Check sheet for the modelled part. Datum: model origin and axes. Units: mm. A direction names the side the tool comes from. Give positions to 0.01 mm unless a question says otherwise; leave off trailing zeros. Order: outer loops, then holes, each group sorted by start corner. A loop starts at its lowest first (then second) coordinate and runs counter-clockwise, first axis right, second up.
Item 1: Sectioned sample at D-D on z = 49. Record the boundary of the cut face in (x, y), and give its area (3 significant figures).
Item 2: Material ranges on line 1 along X through (y, z) = (-24.5, 8); line 2 along Z through (x, y) = (34, -23); line 3 along Z through (x, y) = (18, -21.5), recorded low to high.
Item 3: Gauge pin test, flat ends, axial feed: P1, Ø10, axis at y = -17, z = 9.5, coming from the -X side; P2, Ø6.5, axis at y = -19, z = 34.5, coming from the +X side; P3, Ø5.5, axis at y = -20, z = -6, coming from the -X side; P4, Ø4.5, axis at y = -20.5, z = 8, coming from the -X side. Record the tip position at first contact, or that the pin passes through.
Item 4: Sectioned sample at A-A on z = 9. Record the boundary of the cut face in (x, y), and give its area (3 significant figures).
Item 5: Sectioned sample at B-B on y = -9.5. Record the boundary of the cut face in (x, z), and give its area (3 significant figures).
Item 6: Access from +Z, -Z, +X, -X, +Y, -Y to the whole of each face (thin tool, end or side, straight path). Record for faces 4 (the flat face through (65.827, -19, 27)), 5 (the flat face through (15, -19, 22.991)), 6 (the flat face through (14.111, -19, 1)), 7 (the flat face through (49, -19, 40.581)).
Item 7: Sectioned sample at C-C on x = 49. Record the boundary of the cut face in (y, z).
Item 8: Release check for a two-part mould opening along Z. For faces 1 (the flat face through (40, -6, -15.82)), 2 (the flat face through (31, -19, 40.581)), 3 (the flat face through (52.509, -19, 1)) record: released by +Z, released by -Z, zero draft, split by the parting line, or undercut.
from build123d import *

# Parameters (mm, degrees)
F1_DEPTH = 25.4
F3_DEPTH = 12.7
F4_R     = 3.048


with BuildPart() as f1:
    # F0 (on Front) → F1 (new body)
    with BuildSketch(Plane.XZ):
        Polygon((65.826714, 50.568782), (14.111398, 50.568782), (14.111398, 36.474694), (27.428646, 36.474694), (27.428646, 40.580846), (34.53118, 40.580846), (34.53118, 19.051294), (24.432266, 19.051294), (24.432266, 22.990979), (27.428646, 22.990979), (27.428646, 30.481933), (14.111398, 30.481933), (14.111398, 22.990979), (16.885825, 22.990979), (16.885825, 4.957206), (14.111398, 4.957206), (14.111398, -2.81119), (27.428646, -2.81119), (27.428646, 4.846229), (24.432266, 4.957206), (24.432266, 10.284104), (34.53118, 10.284104), (34.53118, -2.478259), (32.422613, -2.478259), (32.422613, -9.469814), (47.515498, -9.469814), (47.515498, -2.478259), (45.406932, -2.478259), (45.406932, 10.284104), (55.505846, 10.284104), (55.505846, 4.957206), (52.509466, 4.846229), (52.509466, -2.81119), (65.826714, -2.81119), (65.826714, 4.957206), (63.052287, 4.957206), (63.052287, 22.990979), (65.826714, 22.990979), (65.826714, 30.481933), (52.509466, 30.481933), (52.509466, 22.990979), (55.505846, 22.990979), (55.505846, 19.051294), (45.406932, 19.051294), (45.406932, 40.580846), (52.509466, 40.580846), (52.509466, 36.474694), (65.826714, 36.474694), align=None)
    extrude(amount=F1_DEPTH)

    # F2 (on face) → F3 (join)
    with BuildSketch(Plane(origin=(0, 0, 0), x_dir=(-1, 0, 0), z_dir=(0, 1, 0))):
        Polygon((-7.761398, -9.16119), (-7.761398, 56.918782), (-72.176714, 56.918782), (-72.176714, -9.16119), (-53.865498, -9.16119), (-53.865498, -15.819814), (-26.072614, -15.819814), (-26.072614, -9.16119), align=None)
        Polygon((-65.826714, 50.568782), (-14.111398, 50.568782), (-14.111398, 36.474694), (-27.428646, 36.474694), (-27.428646, 40.580846), (-34.53118, 40.580846), (-34.53118, 19.051294), (-24.432266, 19.051294), (-24.432266, 22.990979), (-27.428646, 22.990979), (-27.428646, 30.481933), (-14.111398, 30.481933), (-14.111398, 22.990979), (-16.885825, 22.990979), (-16.885825, 4.957206), (-14.111398, 4.957206), (-14.111398, -2.81119), (-27.428646, -2.81119), (-27.428646, 4.846229), (-24.432266, 4.957206), (-24.432266, 10.284104), (-34.53118, 10.284104), (-34.53118, -2.478259), (-32.422613, -2.478259), (-32.422613, -9.469814), (-47.515498, -9.469814), (-47.515498, -2.478259), (-45.406932, -2.478259), (-45.406932, 10.284104), (-55.505846, 10.284104), (-55.505846, 4.957206), (-52.509466, 4.846229), (-52.509466, -2.81119), (-65.826714, -2.81119), (-65.826714, 4.957206), (-63.052287, 4.957206), (-63.052287, 22.990979), (-65.826714, 22.990979), (-65.826714, 30.481933), (-52.509466, 30.481933), (-52.509466, 22.990979), (-55.505846, 22.990979), (-55.505846, 19.051294), (-45.406932, 19.051294), (-45.406932, 40.580846), (-52.509466, 40.580846), (-52.509466, 36.474694), (-65.826714, 36.474694), align=None, mode=Mode.SUBTRACT)
    extrude(amount=-F3_DEPTH)

    # F4
    f4_edges = [f1.edges().sort_by_distance(p)[0] for p in [
        (7.761398, -6.35, -9.16119),
        (26.072614, -6.35, -9.16119),
        (26.072614, -6.35, -15.819814),
        (53.865498, -6.35, -15.819814),
        (53.865498, -6.35, -9.16119),
        (72.176714, -6.35, -9.16119),
        (72.176714, -6.35, 56.918782),
        (7.761398, -6.35, 56.918782),
    ]]
    fillet(f4_edges, radius=F4_R)


solid = f1.part
Report:
1. outline: (7.76, -12.7) - (14.11, -12.7) - (14.11, -25.4) - (65.83, -25.4) - (65.83, -12.7) - (72.18, -12.7) - (72.18, 0) - (7.76, 0) - close
1. area: 1,470 mm2
2. line 1: x = 16.89 to 24.43, 34.53 to 45.41, 55.51 to 63.05
2. line 2: z = -9.47 to -2.48, 10.28 to 19.05, 40.58 to 50.57
2. line 3: z = -2.81 to 30.48, 36.47 to 50.57
3. P1: stops at x = 7.76
3. P2: stops at x = 65.83
3. P3: stops at x = 32.42
3. P4: stops at x = 16.89
4. outline: (7.76, -12.7) - (16.89, -12.7) - (16.89, -25.4) - (24.43, -25.4) - (24.43, -12.7) - (34.53, -12.7) - (34.53, -25.4) - (45.41, -25.4) - (45.41, -12.7) - (55.51, -12.7) - (55.51, -25.4) - (63.05, -25.4) - (63.05, -12.7) - (72.18, -12.7) - (72.18, 0) - (7.76, 0) - close
4. area: 1,150 mm2
5. outline: (7.76, -6.11) arc R3.05 ccw to (10.81, -9.16) - (23.02, -9.16) arc R3.05 cw to (26.07, -12.21) - (26.07, -12.77) arc R3.05 ccw to (29.12, -15.82) - (50.82, -15.82) arc R3.05 ccw to (53.87, -12.77) - (53.87, -12.21) arc R3.05 cw to (56.91, -9.16) - (69.13, -9.16) arc R3.05 ccw to (72.18, -6.11) - (72.18, 53.87) arc R3.05 ccw to (69.13, 56.92) - (10.81, 56.92) arc R3.05 ccw to (7.76, 53.87) - close
5. area: 4,430 mm2
6. face 4: +Z, -Z, +X, -Y
6. face 5: -X, -Y
6. face 6: +Z, -Z, -X, -Y
6. face 7: -Y
7. outline: (-25.4, 10.28) - (-12.7, 10.28) - (-12.7, -15.82) - (0, -15.82) - (0, 56.92) - (-12.7, 56.92) - (-12.7, 50.57) - (-25.4, 50.57) - (-25.4, 40.58) - (-12.7, 40.58) - (-12.7, 19.05) - (-25.4, 19.05) - close
8. face 1: released by -Z
8. face 2: undercut
8. face 3: zero draft
